from build123d import *

# Parameters (mm, degrees)
F0_W     = 17.2899770278
F0_H     = 12.7
F0_W_2   = 19.05
F0_W_3   = 20.8100229722
F0_H_2   = 9.525
F1_DEPTH = 19.05
F2_R     = 8.89


# Not quite as in the source:
# - a feature names something its author has since deleted; it is built from what else it names


with BuildPart() as f1:
    # F0 (on Front) → F1 (new body)
    with BuildSketch(Plane.XZ):
        with BuildLine():
            Line((-48.4576454937, -259.1044321158), (-48.4576454937, -271.8044321158))
            Line((-48.4576454937, -271.8044321158), (-23.0576454937, -271.8044321158))
            Line((-23.0576454937, -271.8044321158), (-23.0576454937, -259.1044321158))
            Line((-23.0576454937, -259.1044321158), (-23.0576454937, -246.4044321158))
            Line((-23.0576454937, -246.4044321158), (-29.4076454937, -246.4044321158))
            ThreePointArc((-29.4076454937, -246.4044321158), (-35.7576454937, -252.7544321158), (-42.1076454937, -246.4044321158))
            Line((-42.1076454937, -246.4044321158), (-48.4576454937, -246.4044321158))
            Line((-48.4576454937, -246.4044321158), (-48.4576454937, -259.1044321158))
        make_face()
        Polygon((-65.7476225216, -259.1044321158), (-48.4576454937, -271.8044321158), (-48.4576454937, -259.1044321158), align=None)
        Polygon((-23.0576454937, -259.1044321158), (-23.0576454937, -271.8044321158), (-4.0076454937, -259.1044321158), align=None)
        with Locations((-57.1026340077, -252.7544321158)):
            Rectangle(F0_W, F0_H)
        with Locations((-13.5326454937, -252.7544321158)):
            Rectangle(F0_W_2, F0_H)
        with Locations((-57.1026340077, -240.0544321158)):
            Rectangle(F0_W, F0_H)
        with BuildLine():
            Line((-48.4576454937, -233.7044321158), (-48.4576454937, -246.4044321158))
            Line((-48.4576454937, -246.4044321158), (-42.1076454937, -246.4044321158))
            ThreePointArc((-42.1076454937, -246.4044321158), (-35.7576454937, -240.0544321158), (-29.4076454937, -246.4044321158))
            Line((-29.4076454937, -246.4044321158), (-23.0576454937, -246.4044321158))
            Line((-23.0576454937, -246.4044321158), (-23.0576454937, -233.7044321158))
            Line((-23.0576454937, -233.7044321158), (-23.0576454937, -200.7088642316))
            Line((-23.0576454937, -200.7088642316), (-23.0576454937, -168.1484492103))
            Line((-23.0576454937, -168.1484492103), (-23.0576454937, -132.1044321158))
            Line((-23.0576454937, -132.1044321158), (-23.0576454937, -119.4044321158))
            Line((-23.0576454937, -119.4044321158), (-29.4076454937, -119.4044321158))
            ThreePointArc((-29.4076454937, -119.4044321158), (-35.7576454937, -125.7544321158), (-42.1076454937, -119.4044321158))
            Line((-42.1076454937, -119.4044321158), (-48.4576454937, -119.4044321158))
            Line((-48.4576454937, -119.4044321158), (-48.4576454937, -132.1044321158))
            Line((-48.4576454937, -132.1044321158), (-48.4576454937, -168.1484492103))
            Line((-48.4576454937, -168.1484492103), (-48.4576454937, -203.7573134419))
            Line((-48.4576454937, -203.7573134419), (-48.4576454937, -233.7044321158))
        make_face()
        with Locations((-13.5326454937, -240.0544321158)):
            Rectangle(F0_W_2, F0_H)
        Polygon((-65.7476225216, -233.7044321158), (-48.4576454937, -233.7044321158), (-48.4576454937, -203.7573134419), align=None)
        Polygon((-23.0576454937, -200.7088642316), (-23.0576454937, -233.7044321158), (-4.0076454937, -233.7044321158), align=None)
        Polygon((-69.2676684659, -132.1044321158), (-48.4576454937, -168.1484492103), (-48.4576454937, -132.1044321158), align=None)
        Polygon((-23.0576454937, -132.1044321158), (-23.0576454937, -168.1484492103), (-2.2476225216, -132.1044321158), align=None)
        with Locations((-58.8626569798, -125.7544321158)):
            Rectangle(F0_W_3, F0_H)
        with Locations((-12.6526340077, -125.7544321158)):
            Rectangle(F0_W_3, F0_H)
        with Locations((-58.8626569798, -113.0544321158)):
            Rectangle(F0_W_3, F0_H)
        with BuildLine():
            Line((-48.4576454937, -106.7044321158), (-48.4576454937, -119.4044321158))
            Line((-48.4576454937, -119.4044321158), (-42.1076454937, -119.4044321158))
            ThreePointArc((-42.1076454937, -119.4044321158), (-35.7576454937, -113.0544321158), (-29.4076454937, -119.4044321158))
            Line((-29.4076454937, -119.4044321158), (-23.0576454937, -119.4044321158))
            Line((-23.0576454937, -119.4044321158), (-23.0576454937, -106.7044321158))
            Line((-23.0576454937, -106.7044321158), (-23.0576454937, -70.6604150213))
            Line((-23.0576454937, -70.6604150213), (-23.0576454937, 0))
            Line((-23.0576454937, 0), (-23.0576454937, 32.9955678842))
            Line((-23.0576454937, 32.9955678842), (-35.7576454937, 32.9955678842))
            Line((-35.7576454937, 32.9955678842), (-48.4576454937, 32.9955678842))
            Line((-48.4576454937, 32.9955678842), (-48.4576454937, 0))
            Line((-48.4576454937, 0), (-48.4576454937, -70.6604150213))
            Line((-48.4576454937, -70.6604150213), (-48.4576454937, -106.7044321158))
        make_face()
        with Locations((-12.6526340077, -113.0544321158)):
            Rectangle(F0_W_3, F0_H)
        Polygon((-69.2676684659, -106.7044321158), (-48.4576454937, -106.7044321158), (-48.4576454937, -70.6604150213), align=None)
        Polygon((-23.0576454937, -70.6604150213), (-23.0576454937, -106.7044321158), (-2.2476225216, -106.7044321158), align=None)
        Polygon((-67.5076454937, 32.9955678842), (-48.4576454937, 0), (-48.4576454937, 32.9955678842), align=None)
        Polygon((-23.0576454937, 32.9955678842), (-23.0576454937, 0), (-4.0076454937, 32.9955678842), align=None)
        with Locations((-57.9826454937, 37.7580678842)):
            Rectangle(F0_W_2, F0_H_2)
        with Locations((-13.5326454937, 37.7580678842)):
            Rectangle(F0_W_2, F0_H_2)
        with Locations((-57.9826454937, 47.2830678842)):
            Rectangle(F0_W_2, F0_H_2)
        with Locations((-13.5326454937, 47.2830678842)):
            Rectangle(F0_W_2, F0_H_2)
        Polygon((-48.4576454937, 64.7455678842), (-48.4576454937, 52.0455678842), (-35.7576454937, 52.0455678842), (-23.0576454937, 52.0455678842), (-23.0576454937, 64.7455678842), align=None)
        Polygon((-67.5076454937, 52.0455678842), (-48.4576454937, 52.0455678842), (-48.4576454937, 64.7455678842), align=None)
        Polygon((-23.0576454937, 64.7455678842), (-23.0576454937, 52.0455678842), (-4.0076454937, 52.0455678842), align=None)
        with BuildLine():
            Line((-29.4076454937, 42.5205678842), (-23.0576454937, 42.5205678842))
            Line((-23.0576454937, 42.5205678842), (-23.0576454937, 52.0455678842))
            Line((-23.0576454937, 52.0455678842), (-35.7576454937, 52.0455678842))
            Line((-35.7576454937, 52.0455678842), (-35.7576454937, 48.8705678842))
            ThreePointArc((-35.7576454937, 48.8705678842), (-31.2675174332, 47.0106959447), (-29.4076454937, 42.5205678842))
        make_face()
        with BuildLine():
            Line((-48.4576454937, 52.0455678842), (-48.4576454937, 42.5205678842))
            Line((-48.4576454937, 42.5205678842), (-42.1076454937, 42.5205678842))
            ThreePointArc((-42.1076454937, 42.5205678842), (-40.2477735543, 47.0106959447), (-35.7576454937, 48.8705678842))
            Line((-35.7576454937, 48.8705678842), (-35.7576454937, 52.0455678842))
            Line((-35.7576454937, 52.0455678842), (-48.4576454937, 52.0455678842))
        make_face()
        with BuildLine():
            Line((-35.7576454937, 32.9955678842), (-23.0576454937, 32.9955678842))
            Line((-23.0576454937, 32.9955678842), (-23.0576454937, 42.5205678842))
            Line((-23.0576454937, 42.5205678842), (-29.4076454937, 42.5205678842))
            ThreePointArc((-29.4076454937, 42.5205678842), (-31.2675174332, 38.0304398237), (-35.7576454937, 36.1705678842))
            Line((-35.7576454937, 36.1705678842), (-35.7576454937, 32.9955678842))
        make_face()
        with BuildLine():
            Line((-48.4576454937, 42.5205678842), (-48.4576454937, 32.9955678842))
            Line((-48.4576454937, 32.9955678842), (-35.7576454937, 32.9955678842))
            Line((-35.7576454937, 32.9955678842), (-35.7576454937, 36.1705678842))
            ThreePointArc((-35.7576454937, 36.1705678842), (-40.2477735543, 38.0304398237), (-42.1076454937, 42.5205678842))
            Line((-42.1076454937, 42.5205678842), (-48.4576454937, 42.5205678842))
        make_face()
    extrude(amount=F1_DEPTH)

    # F2
    f2_edges = [f1.edges().sort_by_distance(p)[0] for p in [
        (-23.057645, -9.525, -271.804432),
        (-48.457645, -9.525, -271.804432),
    ]]
    fillet(f2_edges, radius=F2_R)


solid = f1.part
Input: part model. Units: mm. Frame: model coordinates. A direction names the side the tool comes from. Coordinates: 2 decimals unless noted, no trailing zeros. Order: outer loops, then holes, each group sorted by start corner. A loop starts at its lowest first (then second) coordinate and runs counter-clockwise, first axis right, second up. Notation, with made-up numbers: M 71,8.5 L 118,8.5 A26 cw 118,36.5 Z; hole C 55.25,74 d9. An arc over 180 degrees is marked long. One line per question, with ' | ' between items.
Item 1: Section B-B (y = -9). Give the number of separate pieces and of enclosed holes in the cut face, then the cut area to 3 significant figures.
Geometry results:
separate pieces: 1 | enclosed holes: 3 | area: 14,000 mm^2
Item 2: Section D-D (z = 11). Output: boundary loops of the cut face in (x, y), then the cut area to 3 significant figures.
Geometry results:
outline: M -54.81,-19.05 L -16.71,-19.05 L -16.71,0 L -54.81,0 Z | area: 726 mm^2
Item 3: Reachability of faces 5 (the flat face through (-4.008, -9, -247)), 6 (the flat face through (-13.666, -9.392, 16.267)), 7 (the flat face through (-67.508, -9, 43)), 8 (the flat face through (-65.748, -9, -246)) from +Z, -Z, +X, -X, +Y, -Y: full face, straight path, thin tool, end or side. Return the list, or none.
Geometry results:
face 5: -Z, +X, +Y, -Y | face 6: +X, +Y, -Y | face 7: +Z, -X, +Y, -Y | face 8: -Z, -X, +Y, -Y
Item 4: Section A-A (x = -18). Output: boundary loops of the cut face in (y, z).
Geometry results:
outline: M -19.05,-268.43 L 0,-268.43 L 0,-209.47 L -19.05,-209.47 Z; M -19.05,-159.39 L 0,-159.39 L 0,-79.42 L -19.05,-79.42 Z; M -19.05,8.76 L 0,8.76 L 0,61.37 L -19.05,61.37 Z
Item 5: Ray query, line 1 along Z through (x, y) = (-62, -9); line 2 along Z through (x, y) = (-64.5, -3); line 3 along Z through (x, y) = (-30.5, -10). Return the intervals inside material, ascending.
Geometry results:
line 1: z = -261.86 to -227.21, -144.69 to -94.12, 23.46 to 55.72 | line 2: z = -260.02 to -231.54, -140.36 to -98.45, 27.79 to 54.05 | line 3: z = -271.8 to -249.97, -242.84 to -122.97, -115.84 to 38.96, 46.08 to 64.75
Item 6: Pin query (flat end, axial travel): pin 1 (9.5 mm diameter, centred on y = -11, z = 38.5, fed in from -X); pin 2 (9.5 mm diameter, centred on y = -5.5, z = -25.5, fed in from -X); pin 3 (3 mm diameter, centred on x = -18.5, y = -2.5, fed in from +Z). Return the tip coordinate at first contact, or that it passes through.
Geometry results:
pin 1: stops at x = -67.51 | pin 2: stops at x = -48.46 | pin 3: stops at z = 62.71
Item 7: Draft query along Z for faces 1 (the flat face through (-69.268, -9, -119)), 2 (the flat face through (-36, -9, 64.746)), 3 (the flat face through (-13.4, -9.39, -217.44)), 4 (the flat face through (-23.058, -9, -185)). Return one class per face: released by +Z, released by -Z, zero draft, split by the parting line, or undercut.
Geometry results:
face 1: zero draft | face 2: released by +Z | face 3: undercut | face 4: undercut
Item 8: Section C-C (z = -250). Output: boundary loops of the cut face in (x, y).
Geometry results:
outline: M -65.75,-19.05 L -40.99,-19.05 L -40.99,0 L -65.75,0 Z; M -30.52,-19.05 L -4.01,-19.05 L -4.01,0 L -30.52,0 Z
